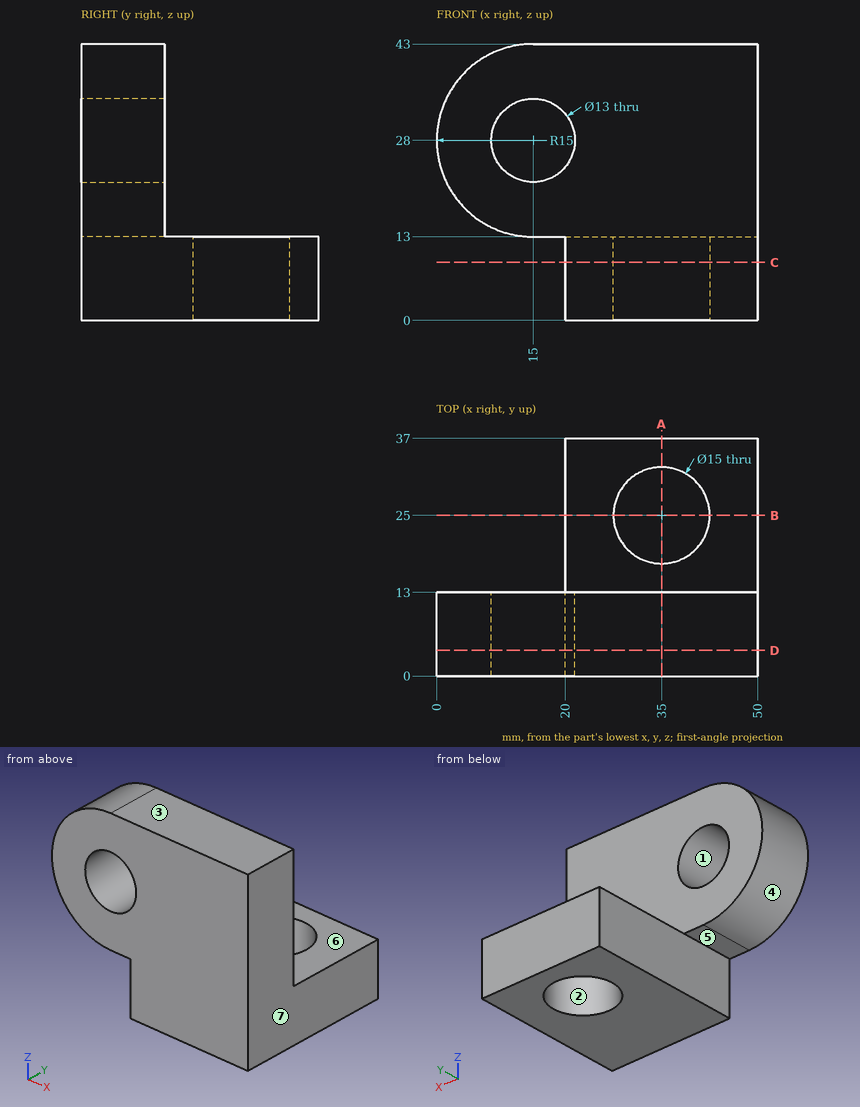
Can you work these out from the drawing? Everything is in mm from the part's minimum corner. A direction names the side the tool comes from. Coordinates: 2 decimals unless noted, no trailing zeros. Loops run counter-clockwise (first coordinate to the right, second up) from the corner with the lowest first, then second, coordinate; pieces in that order, holes last.
1. If we mould it in two halves opening along X, with no side actions, what happens to the marked faces 1, 2, 3 and 4? For each: pulls with the +X half, pulls with the -X half, needs draft (parallel to the pull), parting line crosses it, or undercut.
2. For P1, Ø12, axis at x = 23.5, y = 19.5, coming from the +Z side; P2, Ø17, axis at x = 15, z = 28, coming from the -Y side; P3, Ø6, axis at x = 25, z = 34.5, coming from the +Y side; P4, Ø6.5, axis at y = 11.5, z = 4.5, coming from the -X side, each with a flat end and sliding along its axis, tell me the tip position at first contact or that it passes through.
3. I need wall thicknesses on L1, parallel to Y at x = 35, z = 9.5; L2, parallel to X at y = 8, z = 28; L3, parallel to Y at x = 7, z = 39. Which ranges of each line are inside material? Lowest first, please.
4. Imagine slicing it at A-A, the plane x = 35. Please give me the cut outline in (y, z).
5. For the marked faces 5, 6 and 7, which set-ups out of +Z, -Z, +X, -X, +Y, -Y let a thin tool reach every point of the face, with its end or its side?
6. Imagine slicing it at B-B, the plane y = 25. Please give me the cut outline in (x, z), and give its area (3 significant figures).
7. Imagine slicing it at D-D, the plane y = 4. Please give me the cut outline in (x, z).
8. Imagine slicing it at C-C, the plane z = 9. Please give me the cut outline in (x, y).
Taken from the geometry:
1. face 1: undercut
1. face 2: undercut
1. face 3: needs draft
1. face 4: pulls with the -X half
2. P1: stops at z = 13
2. P2: stops at y = 0
2. P3: stops at y = 13
2. P4: stops at x = 20
3. L1: y = 0 to 17.5, 32.5 to 37
3. L2: x = 0 to 8.5, 21.5 to 50
3. L3: y = 0 to 13
4. outline: (0, 0) - (17.5, 0) - (17.5, 13) - (13, 13) - (13, 43) - (0, 43) - close; (32.5, 0) - (37, 0) - (37, 13) - (32.5, 13) - close
5. face 5: -Z, -X, +Y, -Y
5. face 6: +Z, +X, -X, +Y
5. face 7: +Z, -Z, +X, +Y, -Y
6. outline: (20, 0) - (27.5, 0) - (27.5, 13) - (20, 13) - close; (42.5, 0) - (50, 0) - (50, 13) - (42.5, 13) - close
6. area: 195 mm2
7. outline: (15, 13) - (20, 13) - (20, 0) - (50, 0) - (50, 43) - (15, 43) arc R15 ccw to start; hole circle Ø13 at (15, 28)
8. outline: (20, 0) - (50, 0) - (50, 37) - (20, 37) - close; hole circle Ø15 at (35, 25)
